Job drawing, mm, ordinate dimensions from the low corner. One solid piece. Give positions to 0.01 mm unless a question says otherwise; leave off trailing zeros. Write each loop counter-clockwise with the first axis right and the second up, starting at its lowest first coordinate (ties: lowest second). Pieces come first, ordered by that corner, then holes. Notation, with made-up numbers: (80, 72.5) - (137, 72.5) arc R30 cw to (137, 104.5) - close; hole circle Ø10 at (4.5, 11). An arc over 180 degrees is marked (long way). Answer in a Markdown table with one row per item. Add a question column.
1. Band-saw the part on C-C on z = 40.5. Write the cut outline in (x, y), plus the area to 3 significant figures.
2. Band-saw the part on D-D on x = 30. Write the cut outline in (y, z), plus the area to 3 significant figures.
3. Pull direction X, two halves, no side cores. Call the marked faces 1, 2, 3 and 4: released by +X, released by -X, zero draft, split by the parting line, or undercut.
4. Probe line 1 along Y through (x, z) = (9, 51.75); line 2 along X through (y, z) = (54, 52); line 3 along Y through (x, z) = (30, 59). List the from-to ranges inside material, lowest first.
5. Band-saw the part on B-B on y = 33.5. Write the cut outline in (x, z).
6. Band-saw the part on A-A on z = 48.5. Write the cut outline in (x, y), plus the area to 3 significant figures.
7. Drop flat-ended pins along their axis: pin 1 Ø7 at (x, z) = (30.5, 62) entering from -Y; pin 2 Ø4.5 at (x, z) = (28.5, 7) entering from -Y; pin 3 Ø3 at (x, z) = (47, 25) entering from -Y; pin 4 Ø1.8 at (y, z) = (1, 36) entering from -X. Give the stop position or say it passes through.
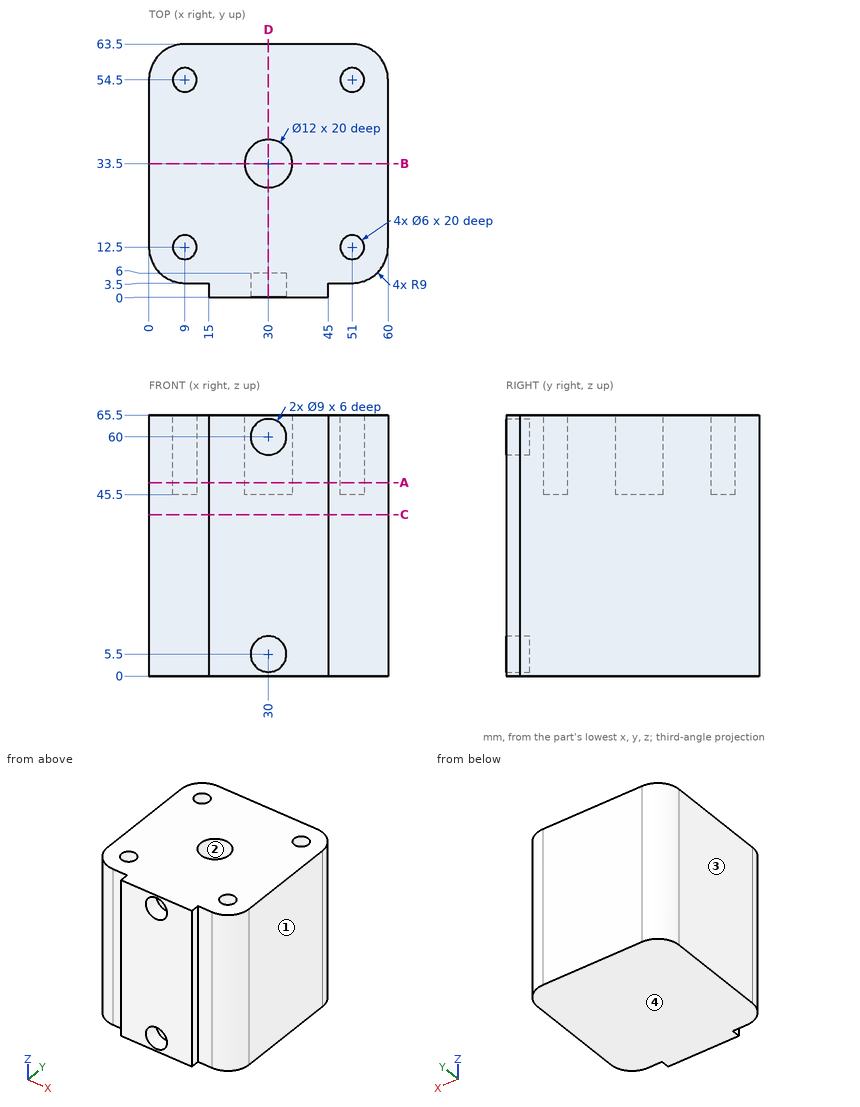
Values:
| question | item | result |
|---|---|---|
| 1 | outline | (0, 12.5) arc R9 ccw to (9, 3.5) - (15, 3.5) - (15, 0) - (45, 0) - (45, 3.5) - (51, 3.5) arc R9 ccw to (60, 12.5) - (60, 54.5) arc R9 ccw to (51, 63.5) - (9, 63.5) arc R9 ccw to (0, 54.5) - close |
| 1 | area | 3,640 mm² |
| 2 | outline | (0, 0) - (63.5, 0) - (63.5, 65.5) - (39.5, 65.5) - (39.5, 45.5) - (27.5, 45.5) - (27.5, 65.5) - (0, 65.5) - (0, 64.5) - (6, 64.5) - (6, 55.5) - (0, 55.5) - (0, 10) - (6, 10) - (6, 1) - (0, 1) - close |
| 2 | area | 3,810 mm² |
| 3 | face 1 | released by +X |
| 3 | face 2 | undercut |
| 3 | face 3 | released by -X |
| 3 | face 4 | zero draft |
| 4 | line 1 | y = 3.5 to 9.5, 15.5 to 51.5, 57.5 to 63.5 |
| 4 | line 2 | x = 0 to 6.04, 11.96 to 48.04, 53.96 to 60 |
| 4 | line 3 | y = 6 to 27.5, 39.5 to 63.5 |
| 5 | outline | (0, 0) - (60, 0) - (60, 65.5) - (36, 65.5) - (36, 45.5) - (24, 45.5) - (24, 65.5) - (0, 65.5) - close |
| 6 | outline | (0, 12.5) arc R9 ccw to (9, 3.5) - (15, 3.5) - (15, 0) - (45, 0) - (45, 3.5) - (51, 3.5) arc R9 ccw to (60, 12.5) - (60, 54.5) arc R9 ccw to (51, 63.5) - (9, 63.5) arc R9 ccw to (0, 54.5) - close; hole circle Ø6 at (9, 12.5); hole circle Ø6 at (9, 54.5); hole circle Ø12 at (30, 33.5); hole circle Ø6 at (51, 12.5); hole circle Ø6 at (51, 54.5) |
| 6 | area | 3,410 mm² |
| 7 | pin 1 | stops at y = 0 |
| 7 | pin 2 | stops at y = 6 |
| 7 | pin 3 | stops at y = 3.5 |
| 7 | pin 4 | stops at x = 15 |
